Verification items for the finished model (mm, model axes). Face numbers are marked on the shaded views. Coordinates: 2 decimals unless noted, no trailing zeros. Loops run counter-clockwise (first coordinate to the right, second up) from the corner with the lowest first, then second, coordinate; pieces in that order, holes last.
Q1. Sectioned sample at C-C (x = 0). Enter the section's corners in (y, z), then the cut area to 3 significant figures.
Q2. Sectioned sample at D-D (x = 75). Enter the section's corners in (y, z).
Q3. Go/stop test with flat-tipped pins: P1, Ø1.9, axis at x = 88.73, z = 13.4, coming from the -Y side; P2, Ø3.5, axis at x = 75, y = 5, coming from the +Z side; P3, Ø2, axis at y = 5, z = 23, coming from the +X side; P4, Ø4, axis at x = 66.51, z = 74.43, coming from the +Y side. Record where each tip stops, or that it passes through.
Q4. Sectioned sample at A-A (x = 43.5). Enter the section's corners in (y, z).
Q5. Mould release check, pull along Z, two halves, no side actions. Record for the marked faces 1 and 2: +Z half, -Z half, draft (parallel to the pull), parting line (faces both ways), or undercut.
Q6. Material ranges on probe 1 along X at (y, z) = (9, 16.5); probe 2 along X at (y, z) = (1.5, 16.5); probe 3 along X at (y, z) = (1.75, 43), recorded low to high.
Q7. Sectioned sample at B-B (z = 30.5). Enter the section's corners in (x, y), then the cut area to 3 significant figures.
```python
from build123d import *

# Parameters (mm, degrees)
MAIN_DEPTH                                     = 10
SKETCH3_R                                      = 1.55
ACTUATOR_SCREW_HOLE_DEPTH                      = 141.91220671
ACTUATOR_SCREW_HOLE_PATTERN_COUNT              = 3
ACTUATOR_SCREW_HOLE_PATTERN_ANGLE              = 80
ACTUATOR_SCREW_HOLE_PATTERN_THE_OTHER_WA_COUNT = 3
ACTUATOR_SCREW_HOLE_PATTERN_THE_OTHER_WA_ANGLE = 80
MIDSPAN_FILLET_R                               = 15
DISH_DEPTH                                     = 5
DISH_FILLET_R                                  = 2.5
F_4_0MM_DOWEL_HOLE1_D                          = 4.1
F_4_0MM_DOWEL_HOLE1_DEPTH                      = 5.7
F_4_0MM_DOWEL_HOLE1_ON_FACE_2_D                = 4.1
F_4_0MM_DOWEL_HOLE1_ON_FACE_2_DEPTH            = 5.7
F_4_0MM_DOWEL_HOLE1_ON_FACE_3_D                = 4.1
F_4_0MM_DOWEL_HOLE1_ON_FACE_3_DEPTH            = 5.7
F_4_0MM_DOWEL_HOLE1_ON_FACE_4_D                = 4.1
F_4_0MM_DOWEL_HOLE1_ON_FACE_4_DEPTH            = 5.7
F_4_0MM_DOWEL_HOLE1_ON_FACE_5_D                = 4.1
F_4_0MM_DOWEL_HOLE1_ON_FACE_5_DEPTH            = 5.7
F_4_0MM_DOWEL_HOLE1_ON_FACE_6_D                = 4.1
F_4_0MM_DOWEL_HOLE1_ON_FACE_6_DEPTH            = 5.7
F_4_0MM_DOWEL_HOLE1_ON_FACE_7_D                = 4.1
F_4_0MM_DOWEL_HOLE1_ON_FACE_7_DEPTH            = 5.7
F_4_0MM_DOWEL_HOLE1_ON_FACE_8_D                = 4.1
F_4_0MM_DOWEL_HOLE1_ON_FACE_8_DEPTH            = 5.7
F_4_0MM_DOWEL_HOLE1_ON_FACE_9_D                = 4.1
F_4_0MM_DOWEL_HOLE1_ON_FACE_9_DEPTH            = 5.7
F_4_0MM_DOWEL_HOLE1_ON_FACE_10_D               = 4.1
F_4_0MM_DOWEL_HOLE1_ON_FACE_10_DEPTH           = 5.7


with BuildPart() as part:
    # Sketch1 → Main (new body)
    with BuildSketch(Plane(origin=(0, 0, 0), x_dir=(1, 0, 0), z_dir=(0, 1, 0))):
        Polygon((0, 12.5), (0, 0), (0, -75), (0, -87.5), (85, -87.5), (110, -62.5), (110, -12.5), (85, 12.5), align=None)
        with BuildLine():
            Line((60, -5), (20, -5))
            Line((20, -5), (20, -70))
            Line((20, -70), (60, -70))
            ThreePointArc((60, -70), (92.5, -37.5), (60, -5))
        make_face(mode=Mode.SUBTRACT)
    extrude(amount=MAIN_DEPTH)

    # Sketch3 → Actuator Screw Hole (cut, through all)
    with BuildSketch(Plane(origin=(0, 10, 0), x_dir=(1, 0, 0), z_dir=(0, 1, 0))):
        with Locations(Location((97.5, -37.5, 0), (0, 0, 270))):
            Circle(SKETCH3_R)
    actuator_screw_hole = extrude(amount=-ACTUATOR_SCREW_HOLE_DEPTH, mode=Mode.SUBTRACT)

    # Actuator Screw Hole Pattern: Actuator Screw Hole ×3 about axis
    actuator_screw_hole_pattern_axis = Axis((60, 0, 37.5), (0, 1, 0))
    for i in range(1, ACTUATOR_SCREW_HOLE_PATTERN_COUNT):
        add(actuator_screw_hole.rotate(actuator_screw_hole_pattern_axis, i * ACTUATOR_SCREW_HOLE_PATTERN_ANGLE / (ACTUATOR_SCREW_HOLE_PATTERN_COUNT - 1)), mode=Mode.SUBTRACT)

    # Actuator Screw Hole Pattern the other wa: Actuator Screw Hole ×3 about axis
    actuator_screw_hole_pattern_the_other_wa_axis = Axis((60, 0, 37.5), (0, -1, 0))
    for i in range(1, ACTUATOR_SCREW_HOLE_PATTERN_THE_OTHER_WA_COUNT):
        add(actuator_screw_hole.rotate(actuator_screw_hole_pattern_the_other_wa_axis, i * ACTUATOR_SCREW_HOLE_PATTERN_THE_OTHER_WA_ANGLE / (ACTUATOR_SCREW_HOLE_PATTERN_THE_OTHER_WA_COUNT - 1)), mode=Mode.SUBTRACT)

    # Midspan fillet
    midspan_fillet_edges = [part.edges().sort_by_distance(p)[0] for p in [
        (20, 5, 5),
        (20, 5, 70),
    ]]
    fillet(midspan_fillet_edges, radius=MIDSPAN_FILLET_R)

    # Mirror1: part across plane


with BuildPart() as part_1:
    add(part.part)
    add(part.part.mirror(Plane(origin=(0, 0, 0), x_dir=(0, 0, 1), z_dir=(1, 0, 0))))

    # Sketch8 → Dish (cut)
    with BuildSketch(Plane(origin=(0, 10, 0), x_dir=(1, 0, 0), z_dir=(0, 1, 0))):
        Polygon((82.100505063, 5.5), (-82.100505063, 5.5), (-103, -15.399494937), (-103, -59.600505063), (-82.100505063, -80.5), (82.100505063, -80.5), (103, -59.600505063), (103, -15.399494937), align=None)
    extrude(amount=-DISH_DEPTH, mode=Mode.SUBTRACT)

    # Dish fillet
    dish_fillet_edges = [part_1.edges().sort_by_distance(p)[0] for p in [
        (92.550252532, 5, 4.949747468),
        (103, 5, 37.5),
        (92.550252532, 5, 70.050252532),
        (0, 5, 80.5),
        (-92.550252532, 5, 70.050252532),
        (-103, 5, 37.5),
        (-92.550252532, 5, 4.949747468),
        (0, 5, -5.5),
    ]]
    fillet(dish_fillet_edges, radius=DISH_FILLET_R)

    # Ø4.0mm Dowel Hole1
    with Locations(Plane(origin=(75, 5, -12.5), x_dir=(-1, 0, 0), z_dir=(0, 0, -1))):
        with Locations((0, 0), (75, 0), (150, 0)):
            Hole(F_4_0MM_DOWEL_HOLE1_D / 2, depth=F_4_0MM_DOWEL_HOLE1_DEPTH)

    # Ø4.0mm Dowel Hole1 on face 2
    with Locations(Plane(origin=(-92.071067812, 5, -5.428932188), x_dir=(-0.707106781187, 0, 0.707106781187), z_dir=(-0.707106781187, 0, -0.707106781187))):
        with Locations((0, 0), (15.355339059, 0)):
            Hole(F_4_0MM_DOWEL_HOLE1_ON_FACE_2_D / 2, depth=F_4_0MM_DOWEL_HOLE1_ON_FACE_2_DEPTH)

    # Ø4.0mm Dowel Hole1 on face 3
    with Locations(Plane(origin=(-110, 5, 22.5), x_dir=(0, 0, -1), z_dir=(-1, 0, 0))):
        with Locations((0, 0), (-30, 0)):
            Hole(F_4_0MM_DOWEL_HOLE1_ON_FACE_3_D / 2, depth=F_4_0MM_DOWEL_HOLE1_ON_FACE_3_DEPTH)

    # Ø4.0mm Dowel Hole1 on face 4
    with Locations(Plane(origin=(-102.928932188, 5, 69.571067812), x_dir=(0.707106781187, 0, 0.707106781187), z_dir=(-0.707106781187, 0, 0.707106781187))):
        with Locations((0, 0)):
            Hole(F_4_0MM_DOWEL_HOLE1_ON_FACE_4_D / 2, depth=F_4_0MM_DOWEL_HOLE1_ON_FACE_4_DEPTH)

    # Ø4.0mm Dowel Hole1 on face 5
    with Locations(Plane(origin=(-92.071067812, 5, 80.428932188), x_dir=(0.707106781187, 0, 0.707106781187), z_dir=(-0.707106781187, 0, 0.707106781187))):
        with Locations((0, 0)):
            Hole(F_4_0MM_DOWEL_HOLE1_ON_FACE_5_D / 2, depth=F_4_0MM_DOWEL_HOLE1_ON_FACE_5_DEPTH)

    # Ø4.0mm Dowel Hole1 on face 6
    with Locations(Plane(origin=(-75, 5, 87.5), x_dir=(1, 0, 0), z_dir=(0, 0, 1))):
        with Locations((0, 0), (75, 0), (150, 0)):
            Hole(F_4_0MM_DOWEL_HOLE1_ON_FACE_6_D / 2, depth=F_4_0MM_DOWEL_HOLE1_ON_FACE_6_DEPTH)

    # Ø4.0mm Dowel Hole1 on face 7
    with Locations(Plane(origin=(92.071067812, 5, 80.428932188), x_dir=(0.707106781187, 0, -0.707106781187), z_dir=(0.707106781187, 0, 0.707106781187))):
        with Locations((0, 0)):
            Hole(F_4_0MM_DOWEL_HOLE1_ON_FACE_7_D / 2, depth=F_4_0MM_DOWEL_HOLE1_ON_FACE_7_DEPTH)

    # Ø4.0mm Dowel Hole1 on face 8
    with Locations(Plane(origin=(102.928932188, 5, 69.571067812), x_dir=(0.707106781187, 0, -0.707106781187), z_dir=(0.707106781187, 0, 0.707106781187))):
        with Locations((0, 0)):
            Hole(F_4_0MM_DOWEL_HOLE1_ON_FACE_8_D / 2, depth=F_4_0MM_DOWEL_HOLE1_ON_FACE_8_DEPTH)

    # Ø4.0mm Dowel Hole1 on face 9
    with Locations(Plane(origin=(110, 5, 52.5), x_dir=(0, 0, 1), z_dir=(1, 0, 0))):
        with Locations((0, 0), (-30, 0)):
            Hole(F_4_0MM_DOWEL_HOLE1_ON_FACE_9_D / 2, depth=F_4_0MM_DOWEL_HOLE1_ON_FACE_9_DEPTH)

    # Ø4.0mm Dowel Hole1 on face 10
    with Locations(Plane(origin=(102.928932188, 5, 5.428932188), x_dir=(-0.707106781187, 0, -0.707106781187), z_dir=(0.707106781187, 0, -0.707106781187))):
        with Locations((0, 0), (15.355339059, 0)):
            Hole(F_4_0MM_DOWEL_HOLE1_ON_FACE_10_D / 2, depth=F_4_0MM_DOWEL_HOLE1_ON_FACE_10_DEPTH)


solid = part_1.part
```
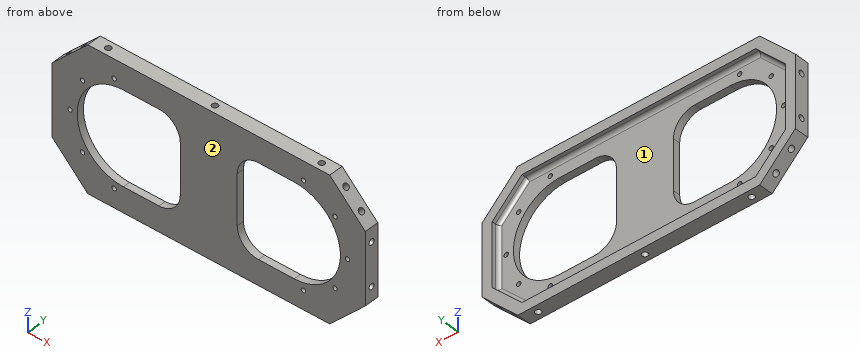
Geometry check:
1. outline: (0, -12.5) - (2.95, -12.5) - (2.95, -6.8) - (7.05, -6.8) - (7.05, -12.5) - (10, -12.5) - (10, -5.5) - (7.5, -5.5) arc R2.5 cw to (5, -3) - (5, 78) arc R2.5 cw to (7.5, 80.5) - (10, 80.5) - (10, 87.5) - (7.05, 87.5) - (7.05, 81.8) - (2.95, 81.8) - (2.95, 87.5) - (0, 87.5) - close
1. area: 526 mm2
2. outline: (0, -12.5) - (2.95, -12.5) - (2.95, -6.8) - (7.05, -6.8) - (7.05, -12.5) - (10, -12.5) - (10, -5.5) - (7.5, -5.5) arc R2.5 cw to (5, -3) - (5, 8.67) - (0, 8.67) - close; (0, 66.33) - (5, 66.33) - (5, 78) arc R2.5 cw to (7.5, 80.5) - (10, 80.5) - (10, 87.5) - (7.05, 87.5) - (7.05, 81.8) - (2.95, 81.8) - (2.95, 87.5) - (0, 87.5) - close
3. P1: passes through
3. P2: stops at z = 81.8
3. P3: stops at x = 104.3
3. P4: stops at y = 5
4. outline: (0, -12.5) - (10, -12.5) - (10, -5.5) - (7.5, -5.5) arc R2.5 cw to (5, -3) - (5, 5) - (0, 5) - close; (0, 70) - (5, 70) - (5, 78) arc R2.5 cw to (7.5, 80.5) - (10, 80.5) - (10, 87.5) - (0, 87.5) - close
5. face 1: undercut
5. face 2: draft
6. probe 1: x = -110 to -103, 103 to 110
6. probe 2: x = -110 to -84.8, -20.41 to 20.41, 84.8 to 110
6. probe 3: x = -110 to -92.03, -20 to 20, 92.03 to 110
7. outline: (-110, 0) - (-91.74, 0) - (-91.74, 5) - (-100.5, 5) arc R2.5 cw to (-103, 7.5) - (-103, 10) - (-110, 10) - close; (-20, 0) - (20, 0) - (20, 5) - (-20, 5) - close; (91.74, 0) - (110, 0) - (110, 10) - (103, 10) - (103, 7.5) arc R2.5 cw to (100.5, 5) - (91.74, 5) - close
7. area: 455 mm2
